Here's how the part is built. I have some questions about the finished solid (model axes, mm). A direction names the side the tool comes from. Coordinates: 2 decimals unless noted, no trailing zeros. Answer as a JSON object with one key per item and string values. Group by question number.
Q1. I'm going to push flat-ended pins straight in: pin 1 (1.5 mm diameter, centred on y = 0, z = 0, fed in from -X); pin 2 (2.5 mm diameter, centred on x = -4.5, y = -4, fed in from +Z); pin 3 (3 mm diameter, centred on x = -3, z = 1.5, fed in from -Y). Where does each tip first touch, or does it pass through?
Q2. On a 3-axis mill with a long thin cutter (end or side, diameter ignored), from which of +Z, -Z, +X, -X, +Y, -Y can I reach the whole of each face in a straight line? I mean faces 4 (the flat face through (-1.829, 0, 0)), 5 (the flat face through (-3, -5.385, -9)). Say none if no direction works.
Q3. Thinking about a two-plate mould opening in Z: for faces 1 (the flat face through (-3, -1, -10.795)), 2 (the flat face through (-6.909, 0, -4)), 3 (the flat face through (-3, -3.099, -5)), which applies, released by +Z, released by -Z, zero draft, split by the parting line, or undercut?
Q4. I need wall thicknesses on line 1 (Z direction, x = -3.45, y = 0) (1 decimal); line 2 (Z direction, x = -5.75, y = -5) (3 decimals); line 3 (Y direction, x = -3, z = -5.5). Which ranges of each line are inside material? Lowest first, please.
Autodesk Fusion 360 part; units mm, degrees
sketch "LegOutline" plane through (0, 0, 0) normal (1, 0, 0) x (0, 1, 0)
  line L0 (3.5052, 0) -> (3.5052, -10.795)
  line L1 (3.5052, -10.795) -> (-5.3848, -10.795)
  line L2 (-5.3848, -10.795) -> (-5.3848, -7.62)
  line L3 (-3.0988, -1.6383) -> (-3.0988, -7.62)
  line L4 (-5.3848, -7.62) -> (-3.0988, -7.62)
  arc A0 (3.5052, 0) -> (-3.0988, -1.6383) centre (0, 0) ccw
  circle A1 centre (0, 0) radius 0.8255
  dimension "d1" = 7.0104
  dimension "d2" = 10.795
  dimension "d3" = 8.89
  dimension "d4" = 3.175
  dimension "d5" = 6.604
  dimension "d6" = 1.651
extrude "Extrude1" add sketch "LegOutline" against normal blind 6.9088 contours L0 L1 L2 L3 L4 A0 | A1
extrude "Extrude2" cut sketch "LegOutline" along normal blind 5.08 from surface at -6.9088 contours A1
fillet "Fillet1" radius 0.0635 2 edges at (-3.4544, -3.0988, -7.62) (-3.4544, -5.3848, -7.62) 3 faces at (-6.9088, 0.236, -6.3945) (0, 1.3039, -6.1383) (-4.6059, 0.5419, -10.795)
Result set:
{
 "1": {"pin 1": "stops at x = -1.83", "pin 2": "stops at z = 2.17", "pin 3": "stops at y = -3.51"},
 "2": {"face 4": "-X", "face 5": "+Z, -Z, +X, -X, -Y"},
 "3": {"face 1": "released by -Z", "face 2": "zero draft", "face 3": "undercut"},
 "4": {"line 1": "z = -10.8 to -0.8, 0.8 to 3.5", "line 2": "z = -10.795 to -7.62", "line 3": "y = -3.1 to 3.51"}
}
